```python
from build123d import *

# Parameters (mm, degrees)
SKETCH1_R           = 25
SKETCH1_R_2         = 4
BOSS_EXTRUDE1_DEPTH = 10
SKETCH2_R           = 5
BOSS_EXTRUDE2_DEPTH = 1
SKETCH3_R           = 4
CUT_EXTRUDE1_DEPTH  = 83


with BuildPart() as part:
    # Sketch1 → Boss-Extrude1 (new body)
    # profile 1 of 2: a face of its own
    with BuildSketch(Plane(origin=(0, 0, 0), x_dir=(1, 0, 0), z_dir=(0, 1, 0))):
        with Locations(Location((0, 0, 0), (0, 0, 270))):
            Circle(SKETCH1_R)
        with BuildLine():
            ThreePointArc((-4.890289414, -10.958333333), (-8.485281374, -8.485281374), (-10.958333333, -4.890289414))
            ThreePointArc((-10.958333333, -4.890289414), (-17, 0), (-10.958333333, 4.890289414))
            ThreePointArc((-10.958333333, 4.890289414), (-8.485281374, 8.485281374), (-4.890289414, 10.958333333))
            ThreePointArc((-4.890289414, 10.958333333), (-0.523714105, 16.97249671), (5, 12))
            ThreePointArc((5, 12), (4.97249671, 11.476285895), (4.890289414, 10.958333333))
            ThreePointArc((4.890289414, 10.958333333), (8.485281374, 8.485281374), (10.958333333, 4.890289414))
            ThreePointArc((10.958333333, 4.890289414), (15.145764348, 3.886407939), (17, 0))
            ThreePointArc((17, 0), (15.145764348, -3.886407939), (10.958333333, -4.890289414))
            ThreePointArc((10.958333333, -4.890289414), (8.485281374, -8.485281374), (4.890289414, -10.958333333))
            ThreePointArc((4.890289414, -10.958333333), (4.97249671, -11.476285895), (5, -12))
            ThreePointArc((5, -12), (-0.523714105, -16.97249671), (-4.890289414, -10.958333333))
        make_face(mode=Mode.SUBTRACT)
    # profile 2 of 2: a face of its own
    with BuildSketch(Plane(origin=(0, 0, 0), x_dir=(1, 0, 0), z_dir=(0, 1, 0))):
        with BuildLine():
            ThreePointArc((-7, 0), (-8.113592061, -3.145764348), (-10.958333333, -4.890289414))
            ThreePointArc((-10.958333333, -4.890289414), (-8.485281374, -8.485281374), (-4.890289414, -10.958333333))
            ThreePointArc((-4.890289414, -10.958333333), (0, -7), (4.890289414, -10.958333333))
            ThreePointArc((4.890289414, -10.958333333), (8.485281374, -8.485281374), (10.958333333, -4.890289414))
            ThreePointArc((10.958333333, -4.890289414), (7, 0), (10.958333333, 4.890289414))
            ThreePointArc((10.958333333, 4.890289414), (8.485281374, 8.485281374), (4.890289414, 10.958333333))
            ThreePointArc((4.890289414, 10.958333333), (0, 7), (-4.890289414, 10.958333333))
            ThreePointArc((-4.890289414, 10.958333333), (-8.485281374, 8.485281374), (-10.958333333, 4.890289414))
            ThreePointArc((-10.958333333, 4.890289414), (-8.113592061, 3.145764348), (-7, 0))
        make_face()
        with Locations(Location((0, 0, 0), (0, 0, 270))):
            Circle(SKETCH1_R_2, mode=Mode.SUBTRACT)
    extrude(amount=BOSS_EXTRUDE1_DEPTH)

    # Sketch2 → Boss-Extrude2 (add)
    with BuildSketch(Plane(origin=(0, 10, 0), x_dir=(1, 0, 0), z_dir=(0, 1, 0))):
        with Locations(Location((0, 0, 0), (0, 0, 270))):
            Circle(SKETCH2_R)
    extrude(amount=BOSS_EXTRUDE2_DEPTH)

    # Sketch3 → Cut-Extrude1 (cut)
    with BuildSketch(Plane.XZ.offset(-10)):
        with Locations(Location((0, 0, 0), (0, 0, 90))):
            Circle(SKETCH3_R)
    extrude(amount=-CUT_EXTRUDE1_DEPTH, mode=Mode.SUBTRACT)


solid = part.part
```
Could you check a few things on this model? Use its own coordinates, in mm. A direction names the side the tool comes from. Give positions to 0.01 mm unless a question says otherwise; leave off trailing zeros. Loops run counter-clockwise (first coordinate to the right, second up) from the corner with the lowest first, then second, coordinate; pieces in that order, holes last. Notation, with made-up numbers: (40, 42.25) - (55, 42.25) arc R23 ccw to (55, 60.25) - close; hole circle Ø5 at (-23.75, 88.25). An arc over 180 degrees is marked (long way). Answer in a Markdown table with one row per item. Add a question column.
Q1. Which directions (+Z, -Z, +X, -X, +Y, -Y) give clear straight access to the entire face, cutting with the end or side of a thin tool? Please do faces 1 (the face through (-4.88, 10.49, -1.08)), 2 (the face through (5, 0, 0)).
Q2. If we section it at C-C (x = 0): List the corners of the cut face in (y, z) for me.
Q3. For pin 1 (1.5 mm diameter, centred on y = 4, z = 9.5, fed in from +X); pin 2 (3 mm diameter, centred on x = -14, y = 2, fed in from -Z); pin 3 (13 mm diameter, centred on x = 0, z = 12, fed in from +Y), each with a flat end and sliding along its axis, tell me the tip position at first contact or that it passes through.
Q4. If we section it at D-D (x = 20): List the corners of the cut face in (y, z) for me.
Q5. If we section it at A-A (x = -15): List the corners of the cut face in (y, z) for me.
Q6. Please list where these lines run through material, in increasing order: L1, parallel to X at y = 7, z = 0; L2, parallel to X at y = 2.5, z = -2.5; L3, parallel to Y at x = 6, z = -19. Write a range as from..to.
Q7. If we section it at B-B (y = 4.75): List the corners of the cut face in (x, z) for me.
The answers:
| question | item | result |
|---|---|---|
| 1 | face 1 | +Y |
| 1 | face 2 | +Z, -Z, +X, -X, -Y |
| 2 | outline | (0, -25) - (10, -25) - (10, -17) - (0, -17) - close; (0, -7) - (10, -7) - (10, -5) - (11, -5) - (11, -4) - (0, -4) - close; (0, 4) - (11, 4) - (11, 5) - (10, 5) - (10, 7) - (0, 7) - close; (0, 17) - (10, 17) - (10, 25) - (0, 25) - close |
| 3 | pin 1 | stops at x = 23.42 |
| 3 | pin 2 | stops at z = -21.65 |
| 3 | pin 3 | stops at y = 10 |
| 4 | outline | (0, -15) - (10, -15) - (10, 15) - (0, 15) - close |
| 5 | outline | (0, -20) - (10, -20) - (10, -4) - (0, -4) - close; (0, 4) - (10, 4) - (10, 20) - (0, 20) - close |
| 6 | L1 | x = -25..-17, -7..-4, 4..7, 17..25 |
| 6 | L2 | x = -24.87..-16.33, -7.67..-3.12, 3.12..7.67, 16.33..24.87 |
| 6 | L3 | y = 0..10 |
| 7 | outline | circle Ø50 at (0, 0); hole circle Ø10 at (-12, 0); hole circle Ø10 at (0, -12); hole circle Ø10 at (0, 12); hole circle Ø8 at (0, 0); hole circle Ø10 at (12, 0) |
